Check sheet for the modelled part. Datum: model origin and axes. Units: mm. Face numbers are marked on the shaded views. A direction names the side the tool comes from. Round coordinates to 2 decimals unless told otherwise and drop trailing zeros. Order: outer loops, then holes, each group sorted by start corner. A loop starts at its lowest first (then second) coordinate and runs counter-clockwise, first axis right, second up.
Q1. Mould release check, pull along X, two halves, no side actions. Record for the marked faces 3, 4 and 5: +X half, -X half, draft (parallel to the pull), parting line (faces both ways), or undercut.
Q2. Depth check by flat-ended pin: P1, Ø2, axis at x = 12, y = 4.5, coming from the -Z side; P2, Ø5, axis at y = 6.5, z = 3.5, coming from the +X side; P3, Ø4, axis at y = -7, z = -5.5, coming from the +X side. Enter the tip coordinate at first touch or a pass-through.
Q3. Set-up check for the marked faces 1 and 2: record each of +Z, -Z, +X, -X, +Y, -Y from which the full face is reachable in a straight line by a thin tool's end or side.
Q4. Cross-section at A-A on y = 0. Record the cut outline in (x, z), then the cut area to 3 significant figures.
Q5. Cross-section at B-B on x = 28. Record the cut outline in (y, z), then the cut area to 3 significant figures.
Q6. Scan lines: probe 1 along X at (y, z) = (5.75, -0.5); probe 2 along Y at (x, z) = (11, -3); probe 3 along Y at (x, z) = (4, -0.75). Record each from-to range of solid material in increasing order.
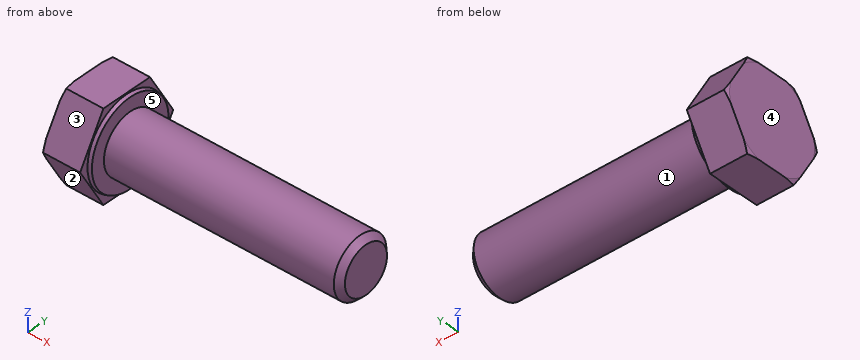
from build123d import *

# Parameters (mm, degrees)
SKETCH_2_OUTSIDE_W  = 30.382
SKETCH_2_OUTSIDE_H  = 30.382
CUT_EXTRUDE_1_DEPTH = 49.811857166
CHAMFER_1_SIZE      = 1


with BuildPart() as part:
    # Эскиз1 → Повернуть1 (revolve)
    with BuildSketch(Plane.XY, mode=Mode.PRIVATE) as revolve_1_sk:
        Polygon((-6.58, 0), (-6.58, 8.85), (0, 8.85), (0, 7.448974596), (0.6, 7.288205081), (0.6, 5), (40.6, 5), (40.6, 0), align=None)
    revolve(revolve_1_sk.sketch.rotate(Axis((-1000, 0, 0), (1, 0, 0)), 90), axis=Axis((-1000, 0, 0), (1, 0, 0)))

    # Эскиз2 outside → Вырез-Вытянуть1 (cut, through all)
    with BuildSketch(Plane.ZY.offset(6.58)):
        Rectangle(SKETCH_2_OUTSIDE_W, SKETCH_2_OUTSIDE_H)
        Polygon((0, -8.85), (7.664324823, -4.425), (7.664324823, 4.425), (0, 8.85), (-7.664324823, 4.425), (-7.664324823, -4.425), align=None, mode=Mode.SUBTRACT)
    extrude(amount=-CUT_EXTRUDE_1_DEPTH, mode=Mode.SUBTRACT)

    # Эскиз4 → Вырез-Повернуть1 (revolve, cut)
    with BuildSketch(Plane.XY):
        Polygon((-6.58, 8.075), (-6.297923068, 8.85), (-6.58, 8.85), align=None)
    revolve(axis=Axis((-1000, 0, 0), (1, 0, 0)), mode=Mode.SUBTRACT)

    # Фаска1
    chamfer_1_edges = [part.edges().sort_by_distance(p)[0] for p in [
        (40.6, 0, -5),
    ]]
    chamfer(chamfer_1_edges, length=CHAMFER_1_SIZE)


solid = part.part
Results found:
1. face 3: draft
1. face 4: -X half
1. face 5: +X half
2. P1: stops at z = -3.57
2. P2: stops at x = 39.72
2. P3: stops at x = 0.6
3. face 1: +X
3. face 2: -Z, +X, -X, -Y
4. outline: (-6.58, -7.66) - (0, -7.66) - (0, -7.45) - (0.6, -7.29) - (0.6, -5) - (39.6, -5) - (40.6, -4) - (40.6, 4) - (39.6, 5) - (0.6, 5) - (0.6, 7.29) - (0, 7.45) - (0, 7.66) - (-6.58, 7.66) - close
4. area: 509 mm2
5. outline: circle Ø10 at (0, 0)
5. area: 78.5 mm2
6. probe 1: x = -6.58 to 0.6
6. probe 2: y = -4 to 4
6. probe 3: y = -4.94 to 4.94
